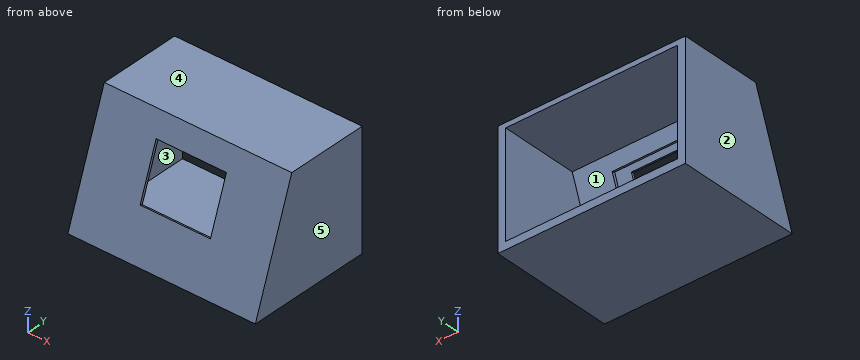
```python
from build123d import *

# Parameters (mm, degrees)
SKETCH003_AS_DRAWN_W                      = 65.558531
SKETCH003_AS_DRAWN_H                      = 42.669216
EXTRUDE002_DEPTH                          = 10
EXTRUDE002_ONTO_SKETCH003_PLACEMENT_ANGLE = 70
EXTRUDE_DEPTH                             = 110
SKETCH001_AS_DRAWN_W                      = 35
SKETCH001_AS_DRAWN_H                      = 45
EXTRUDE001_DEPTH                          = 10
EXTRUDE001_DEPTH_BACK                     = 60
EXTRUDE001_ONTO_SKETCH001_PITCH_ANGLE     = 70
EXTRUDE001_ONTO_SKETCH001_PLACEMENT_ANGLE = -90
PAD_DEPTH                                 = 120


with BuildPart() as extrude002:
    # Sketch003 as drawn → Extrude002 (new)
    with BuildSketch(Plane.XY):
        with Locations((59.320267, 47.473028)):
            Rectangle(SKETCH003_AS_DRAWN_W, SKETCH003_AS_DRAWN_H)
    extrude(amount=EXTRUDE002_DEPTH)


with BuildPart() as extrude002_1:
    # Extrude002 onto Sketch003 placement: moved
    add(extrude002.part.rotate(Axis((0, 0, 0), (1, 0, 0)), EXTRUDE002_ONTO_SKETCH003_PLACEMENT_ANGLE))


with BuildPart() as extrude002_2:
    # Extrude002 placement: moved
    add(extrude002_1.part.moved(Location((0, 11, -4))))


with BuildPart() as extrude_body:
    # Sketch002 (on DatumPlane) → Extrude (new body)
    with BuildSketch(Plane(origin=(120, 0, 120), x_dir=(0, 0, -1), z_dir=(1, 0, 0))):
        Polygon((48.197427, 92.291939), (48.197427, 30.088142), (115.056506, 5.753427), (115.056506, 92.291939), align=None)
    extrude(amount=EXTRUDE_DEPTH)


with BuildPart() as extrude_body_1:
    # Extrude placement: moved
    add(extrude_body.part.moved(Location((-115, 0, 0))))


with BuildPart() as extrude001:
    # Sketch001 as drawn → Extrude001 (new, two sides)
    with BuildSketch(Plane.XY) as extrude001_sk:
        with Locations((-47.5, 60)):
            Rectangle(SKETCH001_AS_DRAWN_W, SKETCH001_AS_DRAWN_H)
    extrude(amount=EXTRUDE001_DEPTH)
    extrude(extrude001_sk.sketch, amount=-EXTRUDE001_DEPTH_BACK)


with BuildPart() as extrude001_1:
    # Extrude001 onto Sketch001 pitch: moved
    add(extrude001.part.rotate(Axis((0, 0, 0), (0, 1, 0)), EXTRUDE001_ONTO_SKETCH001_PITCH_ANGLE))


with BuildPart() as extrude001_2:
    # Extrude001 onto Sketch001 placement: moved
    add(extrude001_1.part.rotate(Axis((0, 0, 0), (0, 0, 1)), EXTRUDE001_ONTO_SKETCH001_PLACEMENT_ANGLE))


with BuildPart() as cut002:
    # Sketch → Pad (new body)
    with BuildSketch(Plane.YZ):
        Polygon((0, 0), (27.297768, 75), (80, 75), (80, 0), align=None)
    extrude(amount=PAD_DEPTH)

    # Cut: cut Extrude001
    add(extrude001_2.part, mode=Mode.SUBTRACT)

    # Cut001: cut Extrude body
    add(extrude_body_1.part, mode=Mode.SUBTRACT)

    # Cut002: cut Extrude002
    add(extrude002_2.part, mode=Mode.SUBTRACT)


solid = cut002.part
```
Could you check a few things on this model? Use its own coordinates, in mm. Face numbers are marked on the shaded views. A direction names the side the tool comes from. Round coordinates to 2 decimals unless told otherwise and drop trailing zeros. Write each loop counter-clockwise with the first axis right and the second up, starting at its lowest first coordinate (ties: lowest second). Pieces come first, ordered by that corner, then holes. Notation, with made-up numbers: M 16.25,70.5 L 38.25,70.5 A20 cw 38.25,98.5 Z; hole C 20.5,26.25 d10. An arc over 180 degrees is marked long. Answer in a Markdown table with one row per item. Add a question column.
Q1. Will these pins go through, and if not, where does the flat tip stop? pin 1 Ø4 at (y, z) = (18.5, 32) entering from -X; pin 2 Ø6 at (x, z) = (24.5, 28.5) entering from -Y; pin 3 Ø5 at (x, z) = (108, 42) entering from -Y; pin 4 Ø5 at (x, z) = (103, 52) entering from +Y.
Q2. If we mould it in two halves opening along X, with no side actions, what happens to the marked faces 3, 4 and 5? For each: +X half, -X half, draft (parallel to the pull), parting line (faces both ways), or undercut.
Q3. Imagine slicing it at C-C (z = 40.5). Please give me the cut outline in (x, y), then the cut area to 3 significant figures.
Q4. If I drill on line 1 (X direction, y = 18, z = 7.5); line 2 (Z direction, x = 98, y = 68.5); line 3 (Z direction, x = 72.5, y = 16), over which ranges is the centre line in solid material (lowest first)? Write a range as from..to.
Q5. Imagine slicing it at B-B (y = 53.5). Please give me the cut outline in (x, z), then the cut area to 3 significant figures.
Q6. On a 3-axis mill with a long thin cutter (end or side, diameter ignored), from which of +Z, -Z, +X, -X, +Y, -Y can I reach the whole of each face in a straight line? I mean the marked faces 1 and 2. Say none if no direction works.
Q7. Imagine slicing it at A-A (x = 56). Please give me the cut outline in (y, z).
Q8. Imagine slicing it at D-D (y = 15). Please give me the cut outline in (x, z), then the cut area to 3 significant figures.
Values:
| question | item | result |
|---|---|---|
| 1 | pin 1 | x = 0 |
| 1 | pin 2 | y = 9.28 |
| 1 | pin 3 | y = 14.38 |
| 1 | pin 4 | y = 23.79 |
| 2 | face 3 | undercut |
| 2 | face 4 | draft |
| 2 | face 5 | +X half |
| 3 | outline | M 0,14.74 L 37.5,14.74 L 37.5,16.55 L 26.54,16.55 L 26.54,18.69 L 5,18.69 L 5,80 L 0,80 Z; M 82.5,14.74 L 120,14.74 L 120,80 L 115,80 L 115,18.69 L 92.1,18.69 L 92.1,16.55 L 82.5,16.55 Z |
| 3 | area | 866 mm^2 |
| 4 | line 1 | 0..5, 115..120 |
| 4 | line 2 | 0..4.94, 71.8..75 |
| 4 | line 3 | 0..4.94 |
| 5 | outline | M 0,0 L 120,0 L 120,75 L 0,75 Z; hole M 5,4.94 L 115,4.94 L 115,71.8 L 5,71.8 Z |
| 5 | area | 1,650 mm^2 |
| 6 | face 1 | +Y |
| 6 | face 2 | +Z, -Z, -X, +Y, -Y |
| 7 | outline | M 0,0 L 80,0 L 80,4.94 L 5.75,4.94 L 12.43,23.29 L 10.54,23.98 L 11.86,27.61 L 10.26,28.19 Z; M 22.23,61.08 L 23.83,60.5 L 25.14,64.08 L 27.03,63.39 L 30.09,71.8 L 80,71.8 L 80,75 L 27.3,75 Z |
| 8 | outline | M 0,0 L 120,0 L 120,41.21 L 82.5,41.21 L 82.5,36.23 L 92.1,36.23 L 92.1,30.35 L 115,30.35 L 115,4.94 L 5,4.94 L 5,30.35 L 26.54,30.35 L 26.54,36.23 L 37.5,36.23 L 37.5,41.21 L 0,41.21 Z |
| 8 | area | 1,540 mm^2 |
